from build123d import *

# Parameters (mm, degrees)
F1_DEPTH = 3.5
F2_W     = 2.45587
F2_H     = 1.399275
F3_DEPTH = 1
F4_R     = 1
F5_R     = 0.3


with BuildPart() as f1:
    # F0 (on Top) → F1 (new body)
    with BuildSketch(Plane.XY):
        Polygon((7.557304, 47.57867), (4.557304, 43.389559), (7.557304, 43.389559), (9.283487, 45.591526), (13.557304, 45.591526), (17.831121, 45.591526), (19.557304, 43.389559), (22.557304, 43.389559), (19.557304, 47.57867), (13.557304, 47.57867), align=None)
    extrude(amount=F1_DEPTH)

    # F2 (on face) → F3 (join)
    with BuildSketch(Plane(origin=(0, 47.57867, 0), x_dir=(-1, 0, 0), z_dir=(0, 1, 0))):
        with Locations((-9.833018, 1.835053)):
            Rectangle(F2_W, F2_H)
    extrude(amount=F3_DEPTH)

    # F4
    f4_edges = [f1.edges().sort_by_distance(p)[0] for p in [
        (7.557304, 47.57867, 1.75),
        (19.557304, 47.57867, 1.75),
    ]]
    fillet(f4_edges, radius=F4_R)

    # F5
    f5_edges = [f1.edges().sort_by_distance(p)[0] for p in [
        (5.907715, 45.275233, 3.5),
        (13.557304, 47.57867, 0),
        (9.833018, 48.57867, 2.534691),
        (11.060953, 48.57867, 1.835054),
        (8.605083, 48.57867, 1.835054),
        (9.833018, 48.57867, 1.135416),
    ]]
    fillet(f5_edges, radius=F5_R)


solid = f1.part
For this review, take the finished solid that the model builds, in its own axes (mm). A direction names the side the tool comes from. Round coordinates to 2 decimals unless told otherwise and drop trailing zeros. Loops run counter-clockwise (first coordinate to the right, second up) from the corner with the lowest first, then second, coordinate; pieces in that order, holes last. Notation, with made-up numbers: (87, 30.25) - (135, 30.25) arc R29 cw to (135, 65.25) - close; hole circle Ø4 at (17, -27.75). An arc over 180 degrees is marked (long way). Put each result on its own line as item: value. Start each with the question number.
1. Consider section B-B on x = 10.25. State the section outline as (y, z) points.
2. For faces 1 (the flat face through (13, 45.592, 2)), 2 (the cylindrical face through (5.96, 45.2, 3.41)), list the 3-axis set-ups (+Z, -Z, +X, -X, +Y, -Y) from which the entire face can be reached by the end or side of a thin tool; tool diameter is ignored.
3. For probe 1 along Y at (x, z) = (11, 0.85); probe 2 along X at (y, z) = (45.2, 0.65); probe 3 along Y at (x, z) = (10.5, 2.15), list the stretches that pass through material, from the lowest coordinate up. Write a range as [from, to].
4. Consider section A-A on z = 2.8. State the section outline as (x, y) points.
5. Insertion check: P1, Ø1.8, axis at x = 13, z = 1.5, coming from the -Y side; P2, Ø2, axis at y = 47, z = 1.5, coming from the -X side; P3, Ø1.5, axis at x = 16.5, z = 2.5, coming from the +Y side. Each pin has a flat end and moves straight along its axis. Give the tip position at first contact, or say it passes through.
6. Consider section C-C on z = 1.6. State the section outline as (x, y) points, plus the area to 3 significant figures.
7. Mouldability with a two-part tool opening along X and no side actions: class faces 3 (the cylindrical face through (21.12, 45.25, 3.41)), 4 (the flat face through (5.927, 45.302, 1.73)), 5 (the flat face through (8.41, 44.48, 1.73)) as +X half, -X half, draft (parallel to the pull), parting line (faces both ways), or undercut.
Result sheet:
1. outline: (45.59, 0) - (47.28, 0) arc R0.3 ccw to (47.58, 0.3) - (47.58, 1.14) - (48.28, 1.14) arc R0.3 ccw to (48.58, 1.44) - (48.58, 2.23) arc R0.3 ccw to (48.28, 2.53) - (47.58, 2.53) - (47.58, 3.2) arc R0.3 ccw to (47.28, 3.5) - (45.59, 3.5) - close
2. face 1: +Z, -Z, -Y
2. face 2: +Z, -X, +Y
3. probe 1: [45.59, 47.58]
3. probe 2: [5.85, 8.98], [18.14, 21.26]
3. probe 3: [45.59, 48.58]
4. outline: (4.56, 43.39) - (7.56, 43.39) - (9.28, 45.59) - (17.83, 45.59) - (19.56, 43.39) - (22.56, 43.39) - (19.86, 47.16) arc R1 ccw to (19.04, 47.58) - (8.07, 47.58) arc R1 ccw to (7.26, 47.16) - close
5. P1: y = 45.59
5. P2: x = 6.43
5. P3: y = 47.58
6. outline: (4.56, 43.39) - (7.56, 43.39) - (9.28, 45.59) - (17.83, 45.59) - (19.56, 43.39) - (22.56, 43.39) - (19.86, 47.16) arc R1 ccw to (19.04, 47.58) - (11.06, 47.58) - (11.06, 48.28) arc R0.3 ccw to (10.76, 48.58) - (8.91, 48.58) arc R0.3 ccw to (8.61, 48.28) - (8.61, 47.58) - (8.07, 47.58) arc R1 ccw to (7.26, 47.16) - close
6. area: 42.6 mm^2
7. face 3: +X half
7. face 4: -X half
7. face 5: undercut
